```python
from build123d import *

# Parameters (mm, degrees)
BOSS_EXTRUDE1_DEPTH = 16
SKETCH3_W           = 56.2
SKETCH3_H           = 30
BOSS_EXTRUDE2_DEPTH = 3
SKETCH4_R           = 1.7
SKETCH4_R_2         = 1.2
CUT_EXTRUDE2_DEPTH  = 19
CUT_EXTRUDE3_DEPTH  = 16
CUT_EXTRUDE6_REACH  = 21
SKETCH10_R          = 2.5
CUT_EXTRUDE7_DEPTH  = 1


with BuildPart() as part:
    # Sketch1 → Boss-Extrude1 (new body)
    with BuildSketch(Plane.XY):
        with BuildLine():
            Line((19.509889407, 0), (0, 0))
            Line((0, 0), (0, -30))
            Line((0, -30), (56.2, -30))
            Line((56.2, -30), (56.2, 0))
            Line((56.2, 0), (36.690110593, 0))
            Line((36.690110593, 0), (35.825930365, 0))
            ThreePointArc((35.825930365, 0), (34.325930365, -1.5), (35.825930365, -3))
            Line((35.825930365, -3), (37.988882647, -3))
            ThreePointArc((37.988882647, -3), (26.465465751, -15.568182447), (19.509889407, 0))
        make_face()
    extrude(amount=BOSS_EXTRUDE1_DEPTH)

    # Sketch3 → Boss-Extrude2 (add)
    with BuildSketch(Plane.XY.offset(16)):
        with Locations((28.1, -15)):
            Rectangle(SKETCH3_W, SKETCH3_H)
    extrude(amount=BOSS_EXTRUDE2_DEPTH)

    # Sketch4 → Cut-Extrude2 (cut)
    with BuildSketch(Plane(origin=(0, 0, 0), x_dir=(-1, 0, 0), z_dir=(0, 0, -1))):
        with Locations((-49.2, -7)):
            Circle(SKETCH4_R)
        with Locations((-7, -7)):
            Circle(SKETCH4_R)
        with Locations((-7, -23)):
            Circle(SKETCH4_R)
        with Locations((-49.2, -23)):
            Circle(SKETCH4_R)
        with Locations((-28.1, -5.5)):
            Circle(SKETCH4_R_2)
    extrude(amount=-CUT_EXTRUDE2_DEPTH, mode=Mode.SUBTRACT)

    # Sketch5 → Cut-Extrude3 (cut)
    with BuildSketch(Plane(origin=(0, 0, 0), x_dir=(-1, 0, 0), z_dir=(0, 0, -1))):
        with BuildLine():
            Line((-19.509889407, 0), (-36.690110593, 0))
            ThreePointArc((-36.690110593, 0), (-28.1, -15.7), (-19.509889407, 0))
        make_face()
    extrude(amount=-CUT_EXTRUDE3_DEPTH, mode=Mode.SUBTRACT)

    # Sketch9 → Cut-Extrude6 (cut, up to next)
    with BuildSketch(Plane.XY, mode=Mode.PRIVATE) as cut_extrude6_sk1:
        with BuildLine():
            Line((36.15, -30), (36.15, -17.197756195))
            ThreePointArc((36.15, -17.197756195), (28.1, -19.7), (20.05, -17.197756195))
            Line((20.05, -17.197756195), (20.05, -30))
            Line((20.05, -30), (36.15, -30))
        make_face()
    cut_extrude6_tool1 = extrude(cut_extrude6_sk1.sketch, amount=CUT_EXTRUDE6_REACH, mode=Mode.PRIVATE) & part.part
    add(cut_extrude6_tool1.solids().sort_by_distance((28.1, -24.424534, 0))[0], mode=Mode.SUBTRACT)

    # Sketch10 → Cut-Extrude7 (cut)
    with BuildSketch(Plane.XY.offset(19)):
        with Locations((28.1, -5.5)):
            Circle(SKETCH10_R)
    extrude(amount=-CUT_EXTRUDE7_DEPTH, mode=Mode.SUBTRACT)


solid = part.part
```
Read the model definition and answer for the solid it produces. Units are mm, in the model's axes. A direction names the side the tool comes from. Round coordinates to 2 decimals unless told otherwise and drop trailing zeros. Write each loop counter-clockwise with the first axis right and the second up, starting at its lowest first coordinate (ties: lowest second). Pieces come first, ordered by that corner, then holes. Notation, with made-up numbers: (22, 58.5) - (50, 58.5) arc R5 ccw to (50, 66.5) - close; hole circle Ø2 at (-12.5, 26.5). An arc over 180 degrees is marked (long way). Use CSV: the item, a comma, the result in double quotes.
Q1. Determine the mould class of faces 1 (the flat face through (28, 0, 18)), 2 (the cylindrical face through (47.63, -7.65, 9.37)), 3 (the flat face through (56.2, -15, 9)) for opening direction X: +X half, -X half, draft (parallel to the pull), parting line (faces both ways), or undercut.
Values:
face 1,"draft"
face 2,"undercut"
face 3,"+X half"
Q2. A tool of negligible diameter and unlimited length cuts with its end or side. For faces 4 (the flat face through (28, -8, 16)), 5 (the cylindrical face through (29.44, -3.39, 18.51)), 6 (the flat face through (10, -30, 9)), 7 (the cylindrical face through (7.221, -21.314, 9.367)), 8 (the flat face through (36.15, -24, 9)), from which of +Z, -Z, +X, -X, +Y, -Y can it reach the whole face along a straight path? Write none if from no direction.
Values:
face 4,"-Z"
face 5,"+Z"
face 6,"+Z, -Z, +X, -X, -Y"
face 7,"+Z, -Z"
face 8,"+Z, -Z, -Y"
Q3. Find section D-D, the plane z = 6.5. Write down the section's boundary in (x, y).
Values:
outline,"(0, -30) - (20.05, -30) - (20.05, -17.2) arc R14.2 ccw to (36.15, -17.2) - (36.15, -30) - (56.2, -30) - (56.2, 0) - (36.69, 0) arc R10.2 cw (long way) to (19.51, 0) - (0, 0) - close; hole circle Ø3.4 at (7, -23); hole circle Ø3.4 at (7, -7); hole circle Ø3.4 at (49.2, -23); hole circle Ø3.4 at (49.2, -7)"
Q4. Find section C-C, the plane x = 49.2. Write down the section's boundary in (y, z).
Values:
outline,"(-30, 0) - (-24.7, 0) - (-24.7, 19) - (-30, 19) - close; (-21.3, 0) - (-8.7, 0) - (-8.7, 19) - (-21.3, 19) - close; (-5.3, 0) - (0, 0) - (0, 19) - (-5.3, 19) - close"
Q5. Find section B-B, the plane y = -23. Write down the section's boundary in (x, z), then the cut area to 3 significant figures.
Values:
outline,"(0, 0) - (5.3, 0) - (5.3, 19) - (0, 19) - close; (8.7, 0) - (20.05, 0) - (20.05, 19) - (8.7, 19) - close; (36.15, 0) - (47.5, 0) - (47.5, 19) - (36.15, 19) - close; (50.9, 0) - (56.2, 0) - (56.2, 19) - (50.9, 19) - close"
area,"633 mm²"
Q6. Find section A-A, the plane x = 28.1. Write down the section's boundary in (y, z), then the cut area to 3 significant figures.
Values:
outline,"(-19.7, 0) - (-15.7, 0) - (-15.7, 16) - (-6.7, 16) - (-6.7, 18) - (-8, 18) - (-8, 19) - (-19.7, 19) - close; (-4.3, 16) - (0, 16) - (0, 19) - (-3, 19) - (-3, 18) - (-4.3, 18) - close"
area,"113 mm²"
Q7. Each of these flat-tipped pins is pushed along its axis until it touches: pin 1 Ø2 at (x, z) = (32.5, 5) entering from +Y; pin 2 Ø8 at (x, y) = (33, -8) entering from -Z; pin 3 Ø2 at (x, z) = (29.5, 8.5) entering from -Y. Where does it stop, or does it pass through?
Values:
pin 1,"stops at y = -14.15"
pin 2,"stops at z = 16"
pin 3,"stops at y = -19.69"
Q8. Straight lines are drawn through the part: line 1 along Y through (x, z) = (7, 13.5); line 2 along X through (y, z) = (-20.75, 14.25). For each, find the intervals that lie inside material, in ascending order.
Values:
line 1,"y = -30 to -24.7, -21.3 to -8.7, -5.3 to 0"
line 2,"x = 0 to 20.05, 36.15 to 56.2"
